Source: CAD feature listing. Evaluate the final solid. Frame: model axes, mm. A direction names the side the tool comes from. Round coordinates to 2 decimals unless told otherwise and drop trailing zeros. Order: outer loops, then holes, each group sorted by start corner. A loop starts at its lowest first (then second) coordinate and runs counter-clockwise, first axis right, second up. Notation, with made-up numbers: (5, 53) - (55, 53) arc R13 cw to (55, 70) - close; hole circle Ø11 at (69.25, -39.5). An arc over 180 degrees is marked (long way). Put each result on its own line as item: value. Start each with the question number.
1) Line query: probe 1 along X at (y, z) = (37, 2); probe 2 along Y at (x, z) = (7, 1); probe 3 along Y at (x, z) = (-6.5, 4.5). Output: solid intervals per line, ascending. Write a range as [from, to].
2) Section B-B on y = 24. Output: boundary loops of the cut face in (x, z).
3) Section A-A on z = 4.75. Output: boundary loops of the cut face in (x, y), then the cut area to 4 significant figures.
4) Access query for faces 4 (the face through (10, 33, 5)), 5 (the face through (50, 1, 5)). Directions: +Z, -Z, +X, -X, +Y, -Y. A direction counts if a zero-diameter tool reaches every point of the face in a straight line with its end or side. Return the directions, or none.
5) Section C-C on x = 8. Output: boundary loops of the cut face in (y, z).
6) Mould query, pull axis X, two halves, no side actions, for faces 1 (the face through (-1, -42.5, 5)), 2 (the face through (-10, 33, 5)), 3 (the face through (-50, 1, 5)). Classes: +X half, -X half, draft (parallel to the pull), parting line (faces both ways), or undercut.
```python
from build123d import *

# Parameters (mm, degrees)
BOSS_EXTRU_1_DEPTH      = 10
ENL_V_MAT_EXTRU_1_DEPTH = 60
BOSS_EXTRU_2_DEPTH      = 40
ESQUISSE5_W             = 10
ESQUISSE5_H             = 30
BOSS_EXTRU_3_DEPTH      = 60
ESQUISSE6_W             = 10
ESQUISSE6_H             = 14
ENL_V_MAT_EXTRU_2_DEPTH = 60
ESQUISSE9_W             = 10
ESQUISSE9_H             = 14
BOSS_EXTRU_4_DEPTH      = 40
ENL_V_MAT_EXTRU_3_DEPTH = 60
BOSS_EXTRU_5_DEPTH      = 40
ESQUISSE13_W            = 10
ESQUISSE13_H            = 31.398637822
BOSS_EXTRU_6_DEPTH      = 60
ENL_V_MAT_EXTRU_9_DEPTH = 60
BOSS_EXTRU_7_DEPTH      = 40


with BuildPart() as part:
    # Esquisse1 → Boss.-Extru.1 (new body)
    with BuildSketch(Plane.XY):
        Polygon((-50, -42.5), (50, -42.5), (50, 42.5), (10, 42.5), (10, 28.5), (0, 28.5), (-10, 28.5), (-10, 42.5), (-50, 42.5), align=None)
    extrude(amount=BOSS_EXTRU_1_DEPTH)

    # Esquisse2 → Enl_v. mat.-Extru.1 (cut)
    with BuildSketch(Plane(origin=(50, 0, 0), x_dir=(0, 0, -1), z_dir=(1, 0, 0))):
        Polygon((-10, 28.5), (0, 18.5), (0, 28.5), align=None)
    extrude(amount=-ENL_V_MAT_EXTRU_1_DEPTH, mode=Mode.SUBTRACT)


with BuildPart() as enl_v_mat_extru_1_piece_1:
    # of the separate pieces the step leaves, piece 1, a body of its own (enl_v_mat_extru_1_pieces)
    add(part.part.solids().sort_by_distance((-50, -42.5, 0))[0])



with BuildPart() as enl_v_mat_extru_1_piece_2:
    # of the separate pieces the step leaves, piece 2, a body of its own (enl_v_mat_extru_1_pieces)
    add(part.part.solids().sort_by_distance((10, 42.5, 10))[0])


with BuildPart() as enl_v_mat_extru_1_piece_1_1:
    add(enl_v_mat_extru_1_piece_1.part)

    add(enl_v_mat_extru_1_piece_2.part)  # Boss.-Extru.2 merges Enl_v. mat.-Extru.1 piece 2
    # Esquisse4 → Boss.-Extru.2 (add)
    with BuildSketch(Plane(origin=(50, 0, 0), x_dir=(0, 0, -1), z_dir=(1, 0, 0))):
        Polygon((-10, 28.5), (0, 18.5), (0, 28.5), align=None)
    extrude(amount=-BOSS_EXTRU_2_DEPTH)

    # Esquisse5 → Boss.-Extru.3 (add)
    with BuildSketch(Plane(origin=(50, 0, 0), x_dir=(0, 0, -1), z_dir=(1, 0, 0))):
        with Locations((-5, 27.5)):
            Rectangle(ESQUISSE5_W, ESQUISSE5_H)
    extrude(amount=-BOSS_EXTRU_3_DEPTH)

    # Esquisse6 → Enl_v. mat.-Extru.2 (cut)
    with BuildSketch(Plane(origin=(50, 0, 0), x_dir=(0, 0, -1), z_dir=(1, 0, 0))):
        with Locations((-5, 35.5)):
            Rectangle(ESQUISSE6_W, ESQUISSE6_H)
    extrude(amount=-ENL_V_MAT_EXTRU_2_DEPTH, mode=Mode.SUBTRACT)

    # Esquisse9 → Boss.-Extru.4 (add)
    with BuildSketch(Plane(origin=(50, 0, 0), x_dir=(0, 0, -1), z_dir=(1, 0, 0))):
        with Locations((-5, 35.5)):
            Rectangle(ESQUISSE9_W, ESQUISSE9_H)
    extrude(amount=-BOSS_EXTRU_4_DEPTH)

    # Esquisse11 → Enl_v. mat.-Extru.3 (cut)
    with BuildSketch(Plane(origin=(50, 0, 0), x_dir=(0, 0, -1), z_dir=(1, 0, 0))):
        Polygon((0, 18.5), (0, 28.5), (-10, 28.5), align=None)
    extrude(amount=-ENL_V_MAT_EXTRU_3_DEPTH, mode=Mode.SUBTRACT)


with BuildPart() as enl_v_mat_extru_3_piece_1:
    # of the separate pieces the step leaves, piece 1, a body of its own (enl_v_mat_extru_3_pieces)
    add(enl_v_mat_extru_1_piece_1_1.part.solids().sort_by_distance((-10, 28.5, 10))[0])



with BuildPart() as enl_v_mat_extru_3_piece_2:
    # of the separate pieces the step leaves, piece 2, a body of its own (enl_v_mat_extru_3_pieces)
    add(enl_v_mat_extru_1_piece_1_1.part.solids().sort_by_distance((10, 42.5, 10))[0])


with BuildPart() as enl_v_mat_extru_3_piece_1_1:
    add(enl_v_mat_extru_3_piece_1.part)

    add(enl_v_mat_extru_3_piece_2.part)  # Boss.-Extru.5 merges Enl_v. mat.-Extru.3 piece 2
    # Esquisse12 → Boss.-Extru.5 (add)
    with BuildSketch(Plane(origin=(50, 0, 0), x_dir=(0, 0, -1), z_dir=(1, 0, 0))):
        Polygon((-10, 28.5), (0, 28.5), (0, 18.5), align=None)
    extrude(amount=-BOSS_EXTRU_5_DEPTH)

    # Esquisse13 → Boss.-Extru.6 (add)
    with BuildSketch(Plane(origin=(50, 0, 0), x_dir=(0, 0, -1), z_dir=(1, 0, 0))):
        with Locations((-5, 12.800681089)):
            Rectangle(ESQUISSE13_W, ESQUISSE13_H)
    extrude(amount=-BOSS_EXTRU_6_DEPTH)

    # Esquisse16 → Enl_v. mat.-Extru.9 (cut)
    with BuildSketch(Plane(origin=(50, 0, 0), x_dir=(0, 0, -1), z_dir=(1, 0, 0))):
        Polygon((-10, 28.5), (0, 28.5), (-10, 18.5), align=None)
    extrude(amount=-ENL_V_MAT_EXTRU_9_DEPTH, mode=Mode.SUBTRACT)


with BuildPart() as enl_v_mat_extru_9_piece_1:
    # of the separate pieces the step leaves, piece 1, a body of its own (enl_v_mat_extru_9_pieces)
    add(enl_v_mat_extru_3_piece_1_1.part.solids().sort_by_distance((50, -42.5, 10))[0])



with BuildPart() as enl_v_mat_extru_9_piece_2:
    # of the separate pieces the step leaves, piece 2, a body of its own (enl_v_mat_extru_9_pieces)
    add(enl_v_mat_extru_3_piece_1_1.part.solids().sort_by_distance((50, 28.5, 10))[0])


with BuildPart() as enl_v_mat_extru_9_piece_1_1:
    add(enl_v_mat_extru_9_piece_1.part)

    add(enl_v_mat_extru_9_piece_2.part)  # Boss.-Extru.7 merges Enl_v. mat.-Extru.9 piece 2
    # Esquisse17 → Boss.-Extru.7 (add)
    with BuildSketch(Plane(origin=(50, 0, 0), x_dir=(0, 0, -1), z_dir=(1, 0, 0))):
        Polygon((-10, 28.5), (0, 28.5), (-10, 18.5), align=None)
    extrude(amount=-BOSS_EXTRU_7_DEPTH)


solid = enl_v_mat_extru_9_piece_1_1.part
```
Answer sheet:
1. probe 1: [-50, -10], [10, 50]
1. probe 2: [-42.5, 27.5]
1. probe 3: [-42.5, 24]
2. outline: (-50, 0) - (50, 0) - (50, 10) - (10, 10) - (10, 4.5) - (-10, 4.5) - (-10, 10) - (-50, 10) - close
3. outline: (-50, -42.5) - (50, -42.5) - (50, 42.5) - (10, 42.5) - (10, 23.75) - (-10, 23.75) - (-10, 42.5) - (-50, 42.5) - close
3. area: 8,125 mm^2
4. face 4: +Z, +Y
4. face 5: +Z, -Z, +X, +Y, -Y
5. outline: (-42.5, 0) - (28.5, 0) - (18.5, 10) - (-42.5, 10) - close
6. face 1: draft
6. face 2: undercut
6. face 3: -X half
